The figure shows three views and two pictorial views of one solid part (mm, origin at its lowest corner). Answer the questions. A direction names the side the tool comes from. Round coordinates to 2 decimals unless told otherwise and drop trailing zeros. Write each loop counter-clockwise with the first axis right and the second up, starting at its lowest first coordinate (ties: lowest second). Pieces come first, ordered by that corner, then holes. Notation, with made-up numbers: M 20.25,-38 L 47.25,-38 A27 cw 47.25,-17 Z; hole C -37.5,48.5 d8. An arc over 180 degrees is marked long. Use one line per item in the form item = value. Start each with the question number.
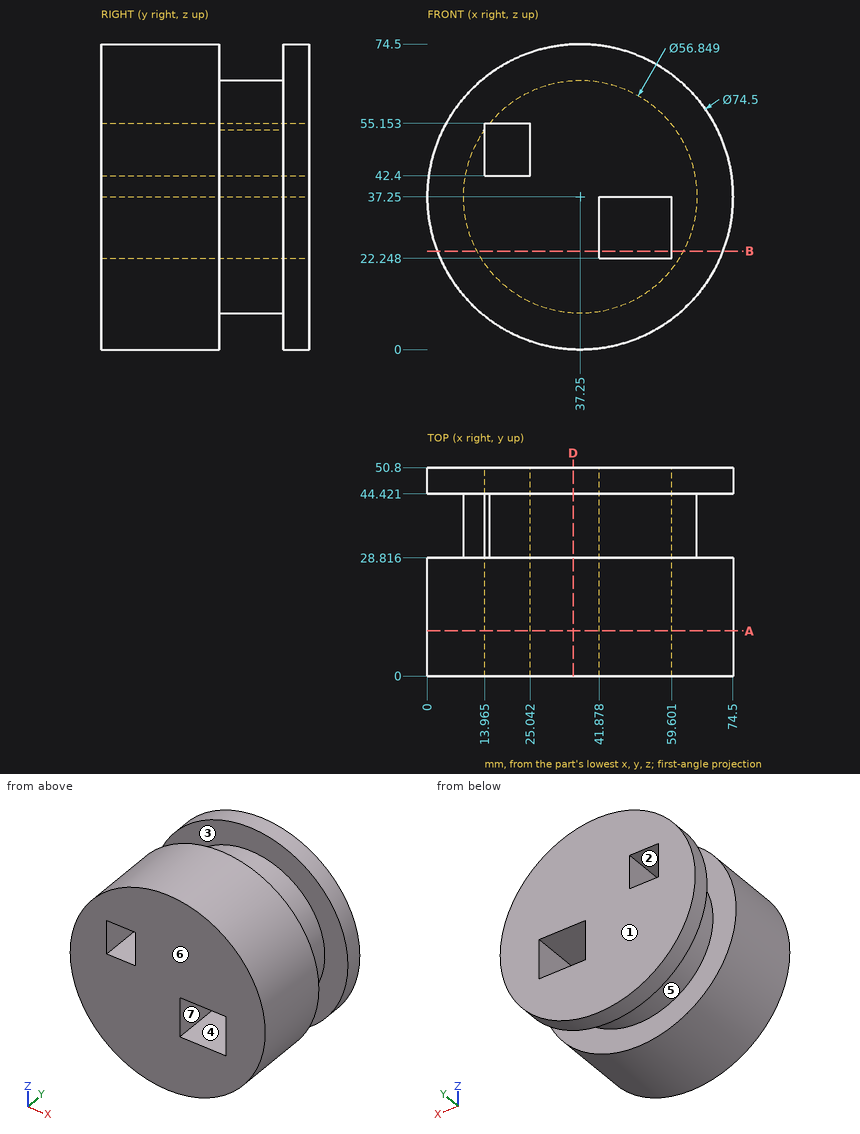
Q1. Find section B-B on z = 24. Write down the section's boundary in (x, y) (1 decimal), and give its area (4 significant figures).
Q2. Find section A-A on y = 11. Count the separate pieces of the cut face and the enclosed holes in it, and give its area (3 significant figures).
Q3. Each of these flat-tipped pins is pushed along its axis until it touches: pin 1 Ø6 at (y, z) = (21, 51) entering from -X (1 decimal); pin 2 Ø1.5 at (y, z) = (22.5, 33.5) entering from +X; pin 3 Ø16.5 at (y, z) = (35, 30) entering from -X. Where does it stop, or does it pass through?
Q4. For a pull along Z with two mould halves and no side action, classify the marked faces 4, 5, 6 and 7 as +Z half, -Z half, draft (parallel to the pull), parting line (faces both ways), or undercut.
Q5. Straight lines are drawn through the part: line 1 (Y direction, x = 21.5, z = 61.5) (1 decimal); line 2 (Z direction, x = 53.5, y = 28.5); line 3 (Z direction, x = 18.5, y = 15.5) (1 decimal). For each, find the intervals that lie inside material, in ascending order. Write a range as [from, to].
Q6. Find section D-D on x = 35.5. Write down the section's boundary in (y, z) (1 decimal).
Q7. A tool of negligible diameter and unlimited length cuts with its end or side. For the marked faces 1, 2 and 3, from which of +Z, -Z, +X, -X, +Y, -Y can it reach the whole face along a straight path? Write none if from no direction.
Response:
q1.outline = M 2.4,0 L 41.9,0 L 41.9,50.8 L 2.4,50.8 L 2.4,44.4 L 12.1,44.4 L 12.1,28.8 L 2.4,28.8 Z; M 59.6,0 L 72.1,0 L 72.1,28.8 L 62.4,28.8 L 62.4,44.4 L 72.1,44.4 L 72.1,50.8 L 59.6,50.8 Z
q1.area = 2,335 mm²
q2.separate_pieces = 1
q2.enclosed_holes = 2
q2.area = 3,950 mm²
q3.pin_1 = 1.6
q3.pin_2 = 74.38
q3.pin_3 = 0.04
q4.face_4 = undercut
q4.face_5 = parting line
q4.face_6 = draft
q4.face_7 = undercut
q5.line_1 = [0, 28.8], [44.4, 50.8]
q5.line_2 = [3.73, 22.25], [37.25, 70.77]
q5.line_3 = [5.1, 42.4], [55.2, 69.4]
q6.outline = M 0,0 L 28.8,0 L 28.8,8.9 L 44.4,8.9 L 44.4,0 L 50.8,0 L 50.8,74.5 L 44.4,74.5 L 44.4,65.6 L 28.8,65.6 L 28.8,74.5 L 0,74.5 Z
q7.face_1 = +Z, -Z, +X, -X, +Y
q7.face_2 = +Y, -Y
q7.face_3 = none
